Source: CAD feature listing. Evaluate the final solid. Frame: model axes, mm. Round coordinates to 2 decimals unless told otherwise and drop trailing zeros. Write each loop counter-clockwise with the first axis right and the second up, starting at its lowest first coordinate (ties: lowest second). Pieces come first, ordered by that corner, then holes. Notation, with made-up numbers: M 12.25,-27 L 27.25,-27 A35 ccw 27.25,5 Z; hole C 65.5,16 d11. An arc over 180 degrees is marked long. Answer in a Markdown table with one row per item. Add a question column.
Item 1: Cut plane A-A on z = 1.2. Return loops of the section in (x, y).
Item 2: Cut plane B-B on y = -93. Return loops of the section in (x, z), and give its area (3 significant figures).
Item 3: Mould query, pull axis Z, two halves, no side actions, for faces 1 (the face through (-3, -244, 0)), 2 (the face through (-3, -244, 2)). Classes: released by +Z, released by -Z, zero draft, split by the parting line, or undercut.
Item 4: Contact query for flat-ended pins moving along their axis: pin 1 (5 mm diameter, centred on x = -168.46, y = -220.46, fed in from -Z); pin 2 (0.6 mm diameter, centred on y = -101, z = 0.5, fed in from -X). Output: stop coordinate, or through.
Item 5: Material intervals for probe 1 along Y at (x, z) = (-181.5, 1.15); probe 2 along Y at (x, z) = (3, 0.7), sorted ascending.
from build123d import *

# Parameters (mm, degrees)
SKETCH1_W           = 400
SKETCH1_H           = 494
BOSS_EXTRUDE1_DEPTH = 2
CUT_EXTRUDE3_DEPTH  = 10
FILLET1_R           = 5
SKETCH6_R           = 2.821572875
CUT_EXTRUDE4_DEPTH  = 60


with BuildPart() as part:
    # Sketch1 → Boss-Extrude1 (new body)
    with BuildSketch(Plane.XY):
        with Locations((0, -247)):
            Rectangle(SKETCH1_W, SKETCH1_H)
    extrude(amount=BOSS_EXTRUDE1_DEPTH)

    # Sketch5 → Cut-Extrude3 (cut)
    with BuildSketch(Plane.XY.offset(2)):
        Polygon((-200, -106), (-200, -79), (-170, -79), (-170, -106), (-170, -131), (-200, -131), align=None)
        Polygon((200, -131), (170, -131), (170, -106), (170, -79), (200, -79), (200, -106), align=None)
    extrude(amount=-CUT_EXTRUDE3_DEPTH, mode=Mode.SUBTRACT)

    # Fillet1
    fillet1_edges = [part.edges().sort_by_distance(p)[0] for p in [
        (-170, -79, 1),
        (-170, -131, 1),
        (170, -131, 1),
        (170, -79, 1),
    ]]
    fillet(fillet1_edges, radius=FILLET1_R)

    # Sketch6 → Cut-Extrude4 (cut)
    with BuildSketch(Plane(origin=(1.544513547, -237.458154074, 2), x_dir=(-1, 0, 0), z_dir=(0, 0, -1))):
        with Locations(Location((-170, 17, 0), (0, 0, 180))):
            Circle(SKETCH6_R)
        with Locations(Location((0, 17, 0), (0, 0, 180))):
            Circle(SKETCH6_R)
        with Locations(Location((170, 17, 0), (0, 0, 180))):
            Circle(SKETCH6_R)
    extrude(amount=CUT_EXTRUDE4_DEPTH, mode=Mode.SUBTRACT)


solid = part.part
Results below:
| question | item | result |
|---|---|---|
| 1 | outline | M -200,-494 L 200,-494 L 200,-131 L 175,-131 A5 cw 170,-126 L 170,-84 A5 cw 175,-79 L 200,-79 L 200,0 L -200,0 L -200,-79 L -175,-79 A5 cw -170,-84 L -170,-126 A5 cw -175,-131 L -200,-131 Z; hole C -168.46,-220.46 d5.64; hole C 1.54,-220.46 d5.64; hole C 171.54,-220.46 d5.64 |
| 2 | outline | M -170,0 L 170,0 L 170,2 L -170,2 Z |
| 2 | area | 680 mm2 |
| 3 | face 1 | released by -Z |
| 3 | face 2 | released by +Z |
| 4 | pin 1 | through |
| 4 | pin 2 | x = -170 |
| 5 | probe 1 | -494 to -131, -79 to 0 |
| 5 | probe 2 | -494 to -222.88, -218.04 to 0 |
